Autodesk Inventor part; units mm, degrees
ref_plane "YZ Plane" through (0, 0, 0) normal (1, 0, 0) x (0, 1, 0)
ref_plane "XZ Plane" through (0, 0, 0) normal (0, 1, 0) x (-1, 0, 0)
ref_plane "XY Plane" through (0, 0, 0) normal (0, 0, 1) x (1, 0, 0)
sketch "Sketch1" plane through (0, 0, 0) normal (0, 0, 1) x (1, 0, 0)
  line L0 (0, 0) -> (50.8, 0)
  line L1 (50.8, 0) -> (50.8, 101.6)
  line L2 (50.8, 101.6) -> (0, 101.6)
  line L3 (0, 101.6) -> (0, 0)
  dimension "d2" = 50.8
  dimension "d3" = 101.6
extrude "Extrusion1" add sketch "Sketch1" along normal blind 1.6
sketch "Sketch2" plane through (0, 0, 1.6) normal (0, 0, 1) x (1, 0, 0)
  line L0 (0, 0) -> (0, 101.6)
  line L1 (50.8, 0) -> (0, 0)
  circle A0 centre (6.35, 12.7) radius 1.6383
  circle A1 centre (6.35, 95.25) radius 1.6383
  circle A2 centre (44.45, 12.7) radius 1.6383
  circle A3 centre (44.45, 95.25) radius 1.6383
  circle A4 centre (37.084, 87.376) radius 0.375
  line L2 (50.8, 101.6) -> (50.8, 0)
  circle A5 centre (39.624, 87.376) radius 0.375
  circle A6 centre (34.544, 87.376) radius 0.375
  dimension "d4" = 3.2766
  dimension "d7" = 82.55
  dimension "d10" = 38.1
  dimension "d13" = 6.35
  dimension "d14" = 12.7
  dimension "d17" = 0.75
  dimension "d20" = 87.376
  dimension "d21" = 13.716
  dimension "d22" = 2.54
  dimension "d23" = 2.54
extrude "Extrusion2" cut sketch "Sketch2" against normal through all
properties part number "circuitBoard"
Input: part model. Units: mm. Frame: model coordinates. Give positions to 0.01 mm unless a question says otherwise; leave off trailing zeros. Loops run counter-clockwise (first coordinate to the right, second up) from the corner with the lowest first, then second, coordinate; pieces in that order, holes last.
1) Section query B-B on x = 6.35. Return the cut outline in (y, z), and give its area (3 significant figures).
A:
outline: (0, 0) - (11.06, 0) - (11.06, 1.6) - (0, 1.6) - close; (14.34, 0) - (93.61, 0) - (93.61, 1.6) - (14.34, 1.6) - close; (96.89, 0) - (101.6, 0) - (101.6, 1.6) - (96.89, 1.6) - close
area: 152 mm2
2) Line query: L1, parallel to Y at x = 44.45, z = 1. Output: solid intervals per line, ascending.
A:
L1: y = 0 to 11.06, 14.34 to 93.61, 96.89 to 101.6
3) Mould query, pull axis Y, two halves, no side actions, for faces 1 (the cylindrical face through (6.137, 96.874, 0.811)), 2 (the flat face through (25, 52, 0)). Classes: released by +Y, released by -Y, zero draft, split by the parting line, or undercut.
A:
face 1: undercut
face 2: zero draft
4) Contact query for a flat-ended pin moving along its axis: pin 1 (5 mm diameter, centred on x = 37.5, y = 49.5, fed in from -Z). Output: stop coordinate, or through.
A:
pin 1: stops at z = 0
5) Section query A-A on y = 12.7. Return the cut outline in (x, z).
A:
outline: (0, 0) - (4.71, 0) - (4.71, 1.6) - (0, 1.6) - close; (7.99, 0) - (42.81, 0) - (42.81, 1.6) - (7.99, 1.6) - close; (46.09, 0) - (50.8, 0) - (50.8, 1.6) - (46.09, 1.6) - close
